```python
from build123d import *

# Parameters (mm, degrees)
SKETCH1_W                    = 193.675
SKETCH1_H                    = 406.4
BOSS_EXTRUDE1_DEPTH          = 1.5875
EDGE_FLANGE1_STRIP_W         = 9.525
EDGE_FLANGE1_STRIP_H         = 1.5875
EDGE_FLANGE1_STRIP_CUT_DEPTH = 193.675
EDGE_FLANGE1_DEPTH           = 193.675
SKETCH5_R                    = 4.2418
CUT_EXTRUDE1_DEPTH           = 2.54


# Sheet-metal steps are written as plain solids
with BuildPart() as part:
    # Sketch1 → Boss-Extrude1 (new body)
    with BuildSketch(Plane.XY):
        with Locations((96.8375, 203.2)):
            Rectangle(SKETCH1_W, SKETCH1_H)
    extrude(amount=BOSS_EXTRUDE1_DEPTH)

    # Edge-Flange1 strip (across the edge) → Edge-Flange1 strip cut (cut)
    with BuildSketch(Plane(origin=(193.675, 406.4, 1.5875), x_dir=(0, -1, 0), z_dir=(-1, 0, 0))):
        with Locations((-1.5875, -0.79375)):
            Rectangle(EDGE_FLANGE1_STRIP_W, EDGE_FLANGE1_STRIP_H)
    extrude(amount=EDGE_FLANGE1_STRIP_CUT_DEPTH, mode=Mode.SUBTRACT)

    # Edge-Flange1 section (across the edge) → Edge-Flange1 (add)
    with BuildSketch(Plane(origin=(193.675, 406.4, 1.5875), x_dir=(0, -1, 0), z_dir=(-1, 0, 0))):
        with BuildLine():
            Line((0, 1.5875), (0, 23.8125))
            Line((0, 23.8125), (1.5875, 23.8125))
            Line((1.5875, 23.8125), (1.5875, 1.5875))
            ThreePointArc((1.5875, 1.5875), (2.052467985, 0.464967985), (3.175, 0))
            Line((3.175, 0), (3.175, -1.5875))
            ThreePointArc((3.175, -1.5875), (0.92993597, -0.65756403), (0, 1.5875))
        make_face()
    extrude(amount=EDGE_FLANGE1_DEPTH)

    # Sketch5 → Cut-Extrude1 (cut)
    with BuildSketch(Plane(origin=(0, 406.4, 0), x_dir=(1, 0, 0), z_dir=(0, 1, 0))):
        with Locations(Location((96.8375, -13.462, 0), (0, 0, 270))):
            Circle(SKETCH5_R)
    extrude(amount=-CUT_EXTRUDE1_DEPTH, mode=Mode.SUBTRACT)


solid = part.part
```
The listing builds one solid part. Answer for the finished solid, in the listing's coordinates (mm). A direction names the side the tool comes from. Give positions to 0.01 mm unless a question says otherwise; leave off trailing zeros. Order: outer loops, then holes, each group sorted by start corner. A loop starts at its lowest first (then second) coordinate and runs counter-clockwise, first axis right, second up. Notation, with made-up numbers: (65.25, -38.5) -> (89.25, -38.5) arc R27 cw to (89.25, -22.5) -> close; hole circle Ø1 at (37, -33). An arc over 180 degrees is marked (long way). Answer as a JSON object with one key per item and string values. Group by question number.
Item 1: Consider L1, parallel to Y at x = 179, z = 19; L2, parallel to Z at x = 116, y = 139.5; L3, parallel to Y at x = 166.5, z = 2.25. Determine where each line is inside the solid, lowest interval first. Write a range as from..to.
Item 2: Determine the mould class of faces 3 (the flat face through (0, 202, 1)), 4 (the flat face through (193.675, 202, 1)), 5 (the flat face through (95, 204, 1.588)), 6 (the cylindrical face through (99.704, 405.617, 10.336)) for opening direction X: pulls with the +X half, pulls with the -X half, needs draft (parallel to the pull), parting line crosses it, or undercut.
Item 3: Flat-ended cylindrical pins translate along their axes: pin 1 (7.5 mm diameter, centred on x = 96.84, z = 13.46, fed in from +Y); pin 2 (4 mm diameter, centred on x = 51, y = 177, fed in from +Z); pin 3 (1.5 mm diameter, centred on x = 99.5, z = 9.5, fed in from -Y). Find the tip coordinate at first contact, or state that the pin passes through.
Item 4: The part is cut by section B-B on z = 13.5. Write down the section's boundary in (x, y) (1 decimal).
Item 5: The part is cut by section C-C on y = 193. Write down the section's boundary in (x, z) (1 decimal), and give its area (3 significant figures).
Item 6: A tool of negligible diameter and unlimited length cuts with its end or side. For faces 1 (the flat face through (95, 204, 0)), 2 (the flat face through (98, 404.812, 19)), from which of +Z, -Z, +X, -X, +Y, -Y can it reach the whole face along a straight path? Write none if from no direction.
Result set:
{
 "1": {"L1": "404.81..406.4", "L2": "0..1.59", "L3": "404.52..406.26"},
 "2": {"face 3": "pulls with the -X half", "face 4": "pulls with the +X half", "face 5": "needs draft", "face 6": "undercut"},
 "3": {"pin 1": "through", "pin 2": "z = 1.59", "pin 3": "y = 404.81"},
 "4": {"outline": "(0, 404.8) -> (92.6, 404.8) -> (92.6, 406.4) -> (0, 406.4) -> close; (101.1, 404.8) -> (193.7, 404.8) -> (193.7, 406.4) -> (101.1, 406.4) -> close"},
 "5": {"outline": "(0, 0) -> (193.7, 0) -> (193.7, 1.6) -> (0, 1.6) -> close", "area": "307 mm²"},
 "6": {"face 1": "-Z, +X, -X, +Y, -Y", "face 2": "+Z, +X, -X, -Y"}
}
